```python
from build123d import *

# Parameters (mm, degrees)
F0_R     = 23.25
F1_DEPTH = 7.7
F5_R     = 7.5
F6_DEPTH = 8.8
F8_DEPTH = 11.601
F9_R     = 3.5
F9_R_2   = 0.25


with BuildPart() as f1:
    # F0 (on Top) → F1 (new body)
    with BuildSketch(Plane.XY):
        Circle(F0_R)
    extrude(amount=F1_DEPTH)

    # F2 (on Front) → F3 (revolve, cut)
    with BuildSketch(Plane.XZ):
        Polygon((17.5, 5.7), (17.5, 11.6), (7.5, 11.6), (0, 11.6), (0, 7.975), align=None)
        Polygon((17.5, 2), (0, 4.275), (0, 0), (0, -2.8375450056), (17.5, -2.8375450056), align=None)
    revolve(axis=Axis((0, 0, 5.8), (0, 0, 1)), mode=Mode.SUBTRACT)

    # F5 (on offset) → F6 (join)
    with BuildSketch(Plane.XY.offset(11.6)):
        Circle(F5_R)
    extrude(amount=-F6_DEPTH)

    # F7 (on offset) → F8 (cut, through all)
    with BuildSketch(Plane.XY.offset(11.6)):
        Polygon((1.025, 3.9692831007), (0, 4.5610671266), (-1.025, 3.9692831007), (-2.925, 2.8723175892), (-3.95, 2.2805335633), (-3.95, 1.0969655115), (-3.95, -1.0969655115), (-3.95, -2.2805335633), (-2.925, -2.8723175892), (-1.025, -3.9692831007), (0, -4.5610671266), (1.025, -3.9692831007), (2.925, -2.8723175892), (3.95, -2.2805335633), (3.95, -1.0969655115), (3.95, 1.0969655115), (3.95, 2.2805335633), (2.925, 2.8723175892), align=None)
        Polygon((-1.025, 3.9692831007), (0, 4.5610671266), (1.025, 3.9692831007), (1.025, 5), (-1.025, 5), align=None)
        Polygon((3.8176270189, 3.3876760389), (2.925, 2.8723175892), (3.95, 2.2805335633), (3.95, 1.0969655115), (4.8426270189, 1.6123239611), align=None)
        Polygon((4.8426270189, -1.6123239611), (3.95, -1.0969655115), (3.95, -2.2805335633), (2.925, -2.8723175892), (3.8176270189, -3.3876760389), align=None)
        Polygon((1.025, -5), (1.025, -3.9692831007), (0, -4.5610671266), (-1.025, -3.9692831007), (-1.025, -5), align=None)
        Polygon((-3.95, -2.2805335633), (-3.95, -1.0969655115), (-4.8426270189, -1.6123239611), (-3.8176270189, -3.3876760389), (-2.925, -2.8723175892), align=None)
        Polygon((-3.95, 2.2805335633), (-2.925, 2.8723175892), (-3.8176270189, 3.3876760389), (-4.8426270189, 1.6123239611), (-3.95, 1.0969655115), align=None)
    extrude(amount=-F8_DEPTH, mode=Mode.SUBTRACT)

    # F9 (on face) → F10 (join, up to the next surface of F1)
    with BuildSketch(Plane.XY.offset(7.7)):
        with Locations((-16, 0)):
            Circle(F9_R)
        with Locations((-16, 0)):
            Circle(F9_R_2, mode=Mode.SUBTRACT)
        with BuildLine():
            ThreePointArc((19.5, 0), (16, 3.5), (12.5, 0))
            ThreePointArc((12.5, 0), (16, -3.5), (19.5, 0))
        make_face()
        with BuildLine():
            ThreePointArc((16.25, 0), (16, -0.25), (15.75, 0))
            ThreePointArc((15.75, 0), (16, 0.25), (16.25, 0))
        make_face(mode=Mode.SUBTRACT)
    extrude(until=Until.NEXT, dir=(0, 0, -1))


solid = f1.part
```
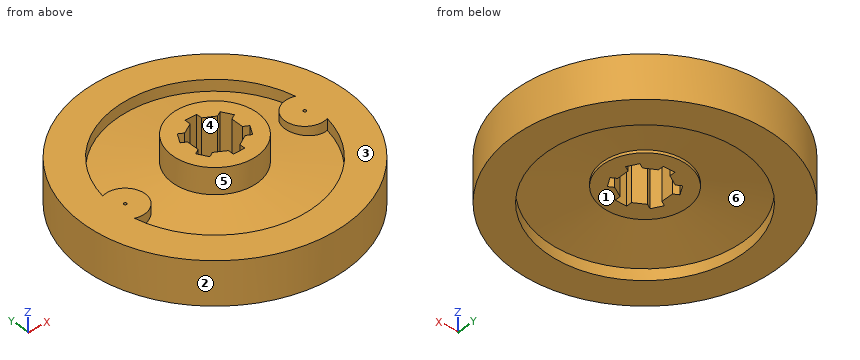
Input: part model. Units: mm. Frame: model coordinates. Face numbers are marked on the shaded views. A direction names the side the tool comes from. Round coordinates to 2 decimals unless told otherwise and drop trailing zeros. Loops run counter-clockwise (first coordinate to the right, second up) from the corner with the lowest first, then second, coordinate; pieces in that order, holes last. Notation, with made-up numbers: (88, 43) -> (126, 43) arc R25 cw to (126, 79) -> close; hole circle Ø1 at (1.25, 47). An arc over 180 degrees is marked (long way). Use one line per item in the form item = value. Start each with the question number.
Item 1: Set-up query: the marked faces 4, 5 and 6. Return all of +Z, -Z, +X, -X, +Y, -Y with unobstructed straight access to the full face (end or side cutting, diameter ignored); none if empty.
Item 2: Mould query, pull axis Y, two halves, no side actions, for the marked faces 1, 2 and 3. Classes: pulls with the +Y half, pulls with the -Y half, needs draft (parallel to the pull), parting line crosses it, or undercut.
Item 3: Section query B-B on z = 1. Return the cut outline in (x, y), then the cut area to 3 significant figures.
Item 4: Section query D-D on x = -19. Return the cut outline in (y, z), then the cut area to 3 significant figures.
Item 5: Section query C-C on y = 20.5. Return the cut outline in (x, z).
Item 6: Contact query for flat-ended pins moving along their axis: pin 1 Ø1.5 at (x, y) = (-5, 11.5) entering from -Z; pin 2 Ø4 at (x, y) = (-3.5, 1) entering from +Z; pin 3 Ø2 at (x, y) = (-17, 1) entering from +Z; pin 4 Ø0.5 at (y, z) = (4.5, 8) entering from -X. Output: stop coordinate, or through.
Item 7: Material intervals for L1, parallel to Y at x = -16, z = 6.6; L2, parallel to Z at x = 19.5, y = -7.5; L3, parallel to Y at x = 0, z = 1.2, sorted ascending. Write a range as from..to.
Item 8: Section query A-A on x = 0. Return the cut outline in (y, z), then the cut area to 3 significant figures.
Ans:
q1.face_4 = +Z, -Z
q1.face_5 = +Z
q1.face_6 = -Z
q2.face_1 = undercut
q2.face_2 = parting line crosses it
q2.face_3 = needs draft
q3.outline = circle Ø46.5 at (0, 0); hole circle Ø35 at (0, 0)
q3.area = 736 mm^2
q4.outline = (-13.4, 0) -> (13.4, 0) -> (13.4, 7.7) -> (-13.4, 7.7) -> close
q4.area = 206 mm^2
q5.outline = (-10.97, 0) -> (10.97, 0) -> (10.97, 7.7) -> (-10.97, 7.7) -> close
q6.pin_1 = 2.55
q6.pin_2 = 11.6
q6.pin_3 = 7.7
q6.pin_4 = -6.18
q7.L1 = -16.87..-7.09, -3.5..-0.25, 0.25..3.5, 7.09..16.87
q7.L2 = 0..7.7
q7.L3 = -23.25..-17.5, 17.5..23.25
q8.outline = (-23.25, 0) -> (-17.5, 0) -> (-17.5, 2) -> (-7.5, 3.3) -> (-7.5, 2.8) -> (-5, 2.8) -> (-5, 11.6) -> (-7.5, 11.6) -> (-7.5, 7) -> (-17.5, 5.7) -> (-17.5, 7.7) -> (-23.25, 7.7) -> close; (5, 2.8) -> (7.5, 2.8) -> (7.5, 3.3) -> (17.5, 2) -> (17.5, 0) -> (23.25, 0) -> (23.25, 7.7) -> (17.5, 7.7) -> (17.5, 5.7) -> (7.5, 7) -> (7.5, 11.6) -> (5, 11.6) -> close
q8.area = 207 mm^2
